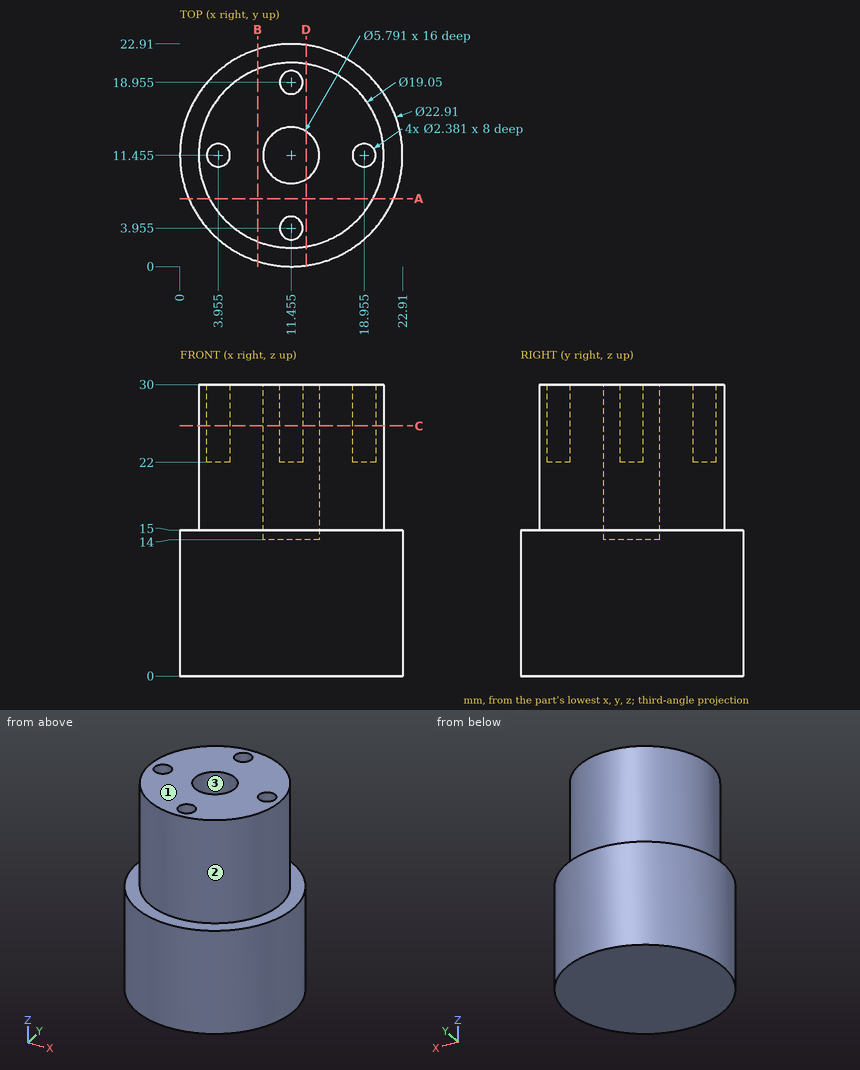
Here's the drawing with two shaded views (mm, measured from the low corner). I have some questions. Give positions to 0.01 mm unless a question says otherwise; leave off trailing zeros. Order: outer loops, then holes, each group sorted by start corner. A loop starts at its lowest first (then second) coordinate and runs counter-clockwise, first axis right, second up. Notation, with made-up numbers: (-11.5, 25) -> (34.5, 25) arc R16 ccw to (34.5, 30) -> close; hole circle Ø8 at (46.5, 81.25). An arc over 180 degrees is marked (long way). One line per item, written item: value. Start each with the question number.
1. Imagine slicing it at C-C, the plane z = 25.75. Count the separate pieces of the cut face and the enclosed holes in it, plus the area to 3 significant figures.
2. Will these pins go through, and if not, where does the flat tip stop? pin 1 Ø4.5 at (x, y) = (11.5, 12) entering from +Z; pin 2 Ø10 at (x, z) = (19.5, 22) entering from -Y; pin 3 Ø1 at (x, z) = (3, 5) entering from +Y.
3. Imagine slicing it at A-A, the plane y = 7. List the corners of the cut face in (x, z) for me, plus the area to 3 significant figures.
4. I need wall thicknesses on probe 1 along X at (y, z) = (12.25, 27.5); probe 2 along X at (y, z) = (11.75, 13.5); probe 3 along Y at (x, z) = (9.5, 26). Which ranges of each line are inside material? Lowest first, please. Write a range as from..to.
5. We'd pull the mould along Y, two halves only. Please class the marked faces 1, 2 and 3: released by +Y, released by -Y, zero draft, split by the parting line, or undercut.
6. Imagine slicing it at B-B, the plane x = 8. List the corners of the cut face in (y, z) for me, plus the area to 3 significant figures.
7. Imagine slicing it at D-D, the plane x = 13. List the corners of the cut face in (y, z) for me (1 decimal).
Values follow:
1. separate pieces: 1
1. enclosed holes: 5
1. area: 241 mm2
2. pin 1: stops at z = 14
2. pin 2: stops at y = 2.43
2. pin 3: stops at y = 19.7
3. outline: (0.9, 0) -> (22.01, 0) -> (22.01, 15) -> (19.87, 15) -> (19.87, 30) -> (3.04, 30) -> (3.04, 15) -> (0.9, 15) -> close
3. area: 569 mm2
4. probe 1: x = 1.96..3.07, 4.84..8.67, 14.24..18.07, 19.84..20.95
4. probe 2: x = 0..22.91
4. probe 3: y = 2.13..9.32, 13.59..20.78
5. face 1: zero draft
5. face 2: split by the parting line
5. face 3: undercut
6. outline: (0.53, 0) -> (22.38, 0) -> (22.38, 15) -> (20.33, 15) -> (20.33, 30) -> (2.58, 30) -> (2.58, 15) -> (0.53, 15) -> close
6. area: 594 mm2
7. outline: (0.1, 0) -> (22.8, 0) -> (22.8, 15) -> (20.9, 15) -> (20.9, 30) -> (13.9, 30) -> (13.9, 14) -> (9, 14) -> (9, 30) -> (2.1, 30) -> (2.1, 15) -> (0.1, 15) -> close
